```python
from build123d import *

# Parameters (mm, degrees)
F3_D     = 13.1064
F2_W     = 6.2990644947
F2_H     = 14.0903731808
F2_W_2   = 3.3267904073
F4_DEPTH = 121.412
F6_DEPTH = 62.23


with BuildPart() as f1:
    # F0 (on Top) → F1 (revolve)
    with BuildSketch(Plane.XY):
        Polygon((-45.5612460607, 0), (0, 0), (0, 41.5925026262), (-45.5612460607, 41.5925026262), (-45.5612460607, 28.2575048772), (-32.8612460607, 28.2575048772), (-32.8612460607, 22.2250052524), (-45.5612460607, 22.2250052524), (-45.5612460607, 15.5575048772), (-30.0037471862, 15.5575048772), (-30.0037471862, 8.5725056276), (-45.5612460607, 8.5725056276), align=None)
    revolve(axis=Axis((0, 20.7962513131, 0), (0, 1, 0)))

    # F3 (through all)
    with Locations(Plane.XZ):
        with Locations((0, 0)):
            Hole(F3_D / 2)

    # F2 (on face) → F4 (cut)
    with BuildSketch(Plane.XZ):
        with BuildLine():
            ThreePointArc((-6.2990644947, 24.6065395066), (0, 25.4), (6.2990644947, 24.6065395066))
            Line((6.2990644947, 24.6065395066), (6.2990644947, 34.3211814761))
            Line((6.2990644947, 34.3211814761), (-6.2990644947, 34.3211814761))
            Line((-6.2990644947, 34.3211814761), (-6.2990644947, 24.6065395066))
        make_face()
        with BuildLine():
            Line((-6.2990644947, -24.6065395066), (-6.2990644947, 24.6065395066))
            ThreePointArc((-6.2990644947, 24.6065395066), (-25.4, 0), (-6.2990644947, -24.6065395066))
        make_face()
        with BuildLine():
            ThreePointArc((6.2990644947, -24.6065395066), (20.0643494557, -15.5750403183), (25.4, 0))
            ThreePointArc((25.4, 0), (20.0643494557, 15.5750403183), (6.2990644947, 24.6065395066))
            Line((6.2990644947, 24.6065395066), (6.2990644947, 14.0903731808))
            Line((6.2990644947, 14.0903731808), (9.625854902, 14.0903731808))
            Line((9.625854902, 14.0903731808), (9.625854902, 0))
            Line((9.625854902, 0), (6.2990644947, 0))
            Line((6.2990644947, 0), (6.2990644947, -24.6065395066))
        make_face()
        with BuildLine():
            Line((6.2990644947, 14.0903731808), (6.2990644947, 24.6065395066))
            ThreePointArc((6.2990644947, 24.6065395066), (0, 25.4), (-6.2990644947, 24.6065395066))
            Line((-6.2990644947, 24.6065395066), (-6.2990644947, -24.6065395066))
            ThreePointArc((-6.2990644947, -24.6065395066), (0, -25.4), (6.2990644947, -24.6065395066))
            Line((6.2990644947, -24.6065395066), (6.2990644947, 0))
            Line((6.2990644947, 0), (0, 0))
            Line((0, 0), (0, 14.0903731808))
            Line((0, 14.0903731808), (6.2990644947, 14.0903731808))
        make_face()
        with Locations((3.1495322473, 7.0451865904)):
            Rectangle(F2_W, F2_H)
        with Locations((7.9624596983, 7.0451865904)):
            Rectangle(F2_W_2, F2_H)
    extrude(amount=-F4_DEPTH, mode=Mode.SUBTRACT)

    # F5 (on face) → F6 (cut)
    with BuildSketch(Plane.XZ):
        with BuildLine():
            ThreePointArc((-2.5140134585, 36.3859235352), (-0.149933756, 36.4723623453), (2.2147767132, 36.4053630567))
            Line((2.2147767132, 36.4053630567), (6.9459112404, 44.897428845))
            ThreePointArc((6.9459112404, 44.897428845), (-0.8987586114, 45.4226488969), (-8.7165118801, 44.5875231483))
            Line((-8.7165118801, 44.5875231483), (-2.5140134585, 36.3859235352))
        make_face()
    extrude(amount=-F6_DEPTH, mode=Mode.SUBTRACT)


solid = f1.part
```
Here's how the part is built. I have some questions about the finished solid (model axes, mm). A direction names the side the tool comes from. Give positions to 0.01 mm unless a question says otherwise; leave off trailing zeros. Write each loop counter-clockwise with the first axis right and the second up, starting at its lowest first coordinate (ties: lowest second). Pieces come first, ordered by that corner, then holes. Notation, with made-up numbers: M -13.5,26 L -6.5,26 A9 cw -6.5,32 Z; hole C 43,89 d2. An arc over 180 degrees is marked long. Put each result on its own line as item: value. Start each with the question number.
Item 1: If we section it at B-B, the plane y = 13: Write out the boundary of the cut face in (x, z).
Item 2: If we section it at A-A, the plane z = 22.5: Write out the boundary of the cut face in (x, y) (1 decimal), then the cut area to 3 significant figures.
Item 3: If we section it at C-C, the plane x = 35: Write out the boundary of the cut face in (y, z) (1 decimal).
Item 4: On a 3-axis mill with a long thin cutter (end or side, diameter ignored), from which of +Z, -Z, +X, -X, +Y, -Y can I reach the whole of each face in a straight line? I mean faces 5 (the flat face through (20, 41.593, -20)), 6 (the flat face through (14, 28.258, -30)), 7 (the flat face through (6.299, 21, 29)). Say none if no direction works.
Item 5: Will these pins go through, and if not, where does the flat tip stop? pin 1 (1 mm diameter, centred on y = 22, z = 15, fed in from +X); pin 2 (5 mm diameter, centred on y = 30, z = 29.5, fed in from +X); pin 3 (5 mm diameter, centred on x = -27.5, y = 32.5, fed in from +Z).
Item 6: I need wall thicknesses on L1, parallel to Y at x = 2.5, z = -38 (1 decimal); L2, parallel to X at y = 20, z = 15; L3, parallel to Z at x = -9, y = 38. Which ranges of each line are inside material? Lowest first, please. Write a range as from..to.
Item 7: Thinking about a two-plate mould opening in Y: for faces 1 (the cylindrical face through (1.23, 12.02, -29.98)), 2 (the flat face through (-20, 0, -20)), 3 (the flat face through (-9, 15.558, -30)), 4 (the cylindrical face through (-0.183, 4.226, 36.472)), which applies, +Y half, -Y half, draft (parallel to the pull), parting line (faces both ways), or undercut?
Item 8: If we section it at D-D, the plane y = 34.5: Write out the boundary of the cut face in (x, z), then the cut area to 3 significant figures.
Values:
1. outline: M -6.3,24.61 L -6.3,29.34 A30 ccw long 6.3,29.34 L 6.3,24.61 A25.4 cw long Z
2. outline: M -39.6,0 L -11.8,0 L -11.8,41.6 L -39.6,41.6 L -39.6,28.3 L -24,28.3 L -24,22.2 L -39.6,22.2 L -39.6,15.6 L -19.8,15.6 L -19.8,8.6 L -39.6,8.6 Z; M 11.8,0 L 39.6,0 L 39.6,8.6 L 19.8,8.6 L 19.8,15.6 L 39.6,15.6 L 39.6,22.2 L 24,22.2 L 24,28.3 L 39.6,28.3 L 39.6,41.6 L 11.8,41.6 Z
2. area: 1,850 mm²
3. outline: M 0,-29.2 L 8.6,-29.2 L 8.6,29.2 L 0,29.2 Z; M 15.6,-29.2 L 22.2,-29.2 L 22.2,29.2 L 15.6,29.2 Z; M 28.3,-29.2 L 41.6,-29.2 L 41.6,29.2 L 28.3,29.2 Z
4. face 5: +Z, -Z, +X, -X, +Y
4. face 6: none
4. face 7: +Y, -Y
5. pin 1: x = 43.19
5. pin 2: x = 36.7
5. pin 3: z = 38.09
6. L1: 0..8.6, 15.6..22.2, 28.3..41.6
6. L2: -43.02..-20.5, 20.5..43.02
6. L3: -44.66..-23.75, 23.75..44.66
7. face 1: undercut
7. face 2: -Y half
7. face 3: undercut
7. face 4: draft
8. outline: C 0,0 d91.12; hole M -8.72,44.59 L -2.51,36.39 A36.47 cw 2.21,36.41 L 6.95,44.9 A45.43 ccw Z; hole M -6.3,24.61 A25.4 ccw long 6.3,24.61 L 6.3,34.32 L -6.3,34.32 Z
8. area: 4,290 mm²
